Read the model definition and answer for the solid it produces. Units are mm, in the model's axes. Give positions to 0.01 mm unless a question says otherwise; leave off trailing zeros. Loops run counter-clockwise (first coordinate to the right, second up) from the corner with the lowest first, then second, coordinate; pieces in that order, holes last. Notation, with made-up numbers: M 11.5,-6 L 24.5,-6 A29 cw 24.5,24 Z; hole C 60.5,77.25 d9. An arc over 180 degrees is marked long. Return JSON: item names as keys, results as strings. Group by question number.
```python
from build123d import *

# Parameters (mm, degrees)
SKETCH1_W           = 92
SKETCH1_H           = 50
SKETCH1_R           = 10.5
SKETCH1_R_2         = 1.55
BOSS_EXTRUDE1_DEPTH = 3
FILLET1_R           = 4
SKETCH_1_R          = 3.05
CUT_EXTRUDE_1_DEPTH = 10


with BuildPart() as part:
    # Sketch1 → Boss-Extrude1 (new body)
    with BuildSketch(Plane(origin=(0, 0, 0), x_dir=(1, 0, 0), z_dir=(0, 1, 0))):
        Rectangle(SKETCH1_W, SKETCH1_H)
        with Locations(Location((0, 0, 0), (0, 0, 270))):
            Circle(SKETCH1_R, mode=Mode.SUBTRACT)
        with Locations(Location((42, 21, 0), (0, 0, 270))):
            Circle(SKETCH1_R_2, mode=Mode.SUBTRACT)
        with Locations(Location((-42, 21, 0), (0, 0, 90))):
            Circle(SKETCH1_R_2, mode=Mode.SUBTRACT)
        with Locations(Location((42, -21, 0), (0, 0, 90))):
            Circle(SKETCH1_R_2, mode=Mode.SUBTRACT)
        with Locations(Location((-42, -21, 0), (0, 0, 270))):
            Circle(SKETCH1_R_2, mode=Mode.SUBTRACT)
        with Locations(Location((0, -18, 0), (0, 0, 270))):
            Circle(SKETCH1_R_2, mode=Mode.SUBTRACT)
        with Locations(Location((-15.588457268, 9, 0), (0, 0, 270))):
            Circle(SKETCH1_R_2, mode=Mode.SUBTRACT)
        with Locations(Location((15.588457268, 9, 0), (0, 0, 270))):
            Circle(SKETCH1_R_2, mode=Mode.SUBTRACT)
    extrude(amount=BOSS_EXTRUDE1_DEPTH)

    # Fillet1
    fillet1_edges = [part.edges().sort_by_distance(p)[0] for p in [
        (46, 1.5, 25),
        (-46, 1.5, 25),
        (-46, 1.5, -25),
        (46, 1.5, -25),
    ]]
    fillet(fillet1_edges, radius=FILLET1_R)

    # 草图1 → 切除-拉伸1 (cut)
    with BuildSketch(Plane.XZ):
        with Locations(Location((-22.5, 0, 0), (0, 0, 270))):
            Circle(SKETCH_1_R)
        with Locations(Location((22.5, 0, 0), (0, 0, 270))):
            Circle(SKETCH_1_R)
    extrude(amount=-CUT_EXTRUDE_1_DEPTH, mode=Mode.SUBTRACT)


solid = part.part
```
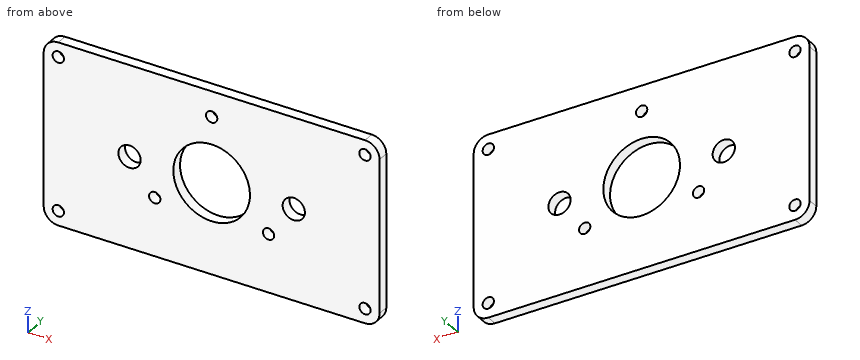
1. A flat-ended cylindrical pin translates along its axis: P1, Ø3, axis at x = 42, z = 21, coming from the +Y side. Find the tip coordinate at first contact, or state that the pin passes through.
2. Straight lines are drawn through the part: line 1 along X through (y, z) = (1.45, -21); line 2 along X through (y, z) = (1.5, -9); line 3 along X through (y, z) = (0.7, -2). For each, find the intervals that lie inside material, in ascending order.
3. Find section B-B (x = 22.5). Write down the section's boundary in (y, z), and give its area (3 significant figures).
4. Find section C-C (z = 0). Write down the section's boundary in (x, y), and give its area (3 significant figures).
5. Find section D-D (y = 0.85). State how many separate pieces and enclosed holes the cut face has, and give its area (3 significant figures).
6. Find section A-A (z = 18). Write down the section's boundary in (x, y).
Result:
{
 "1": {"P1": "passes through"},
 "2": {"line 1": "x = -46 to -43.55, -40.45 to 40.45, 43.55 to 46", "line 2": "x = -46 to -17.14, -14.04 to -5.41, 5.41 to 14.04, 17.14 to 46", "line 3": "x = -46 to -24.8, -20.2 to -10.31, 10.31 to 20.2, 24.8 to 46"},
 "3": {"outline": "M 0,-25 L 3,-25 L 3,-3.05 L 0,-3.05 Z; M 0,3.05 L 3,3.05 L 3,25 L 0,25 Z", "area": "132 mm2"},
 "4": {"outline": "M -46,0 L -25.55,0 L -25.55,3 L -46,3 Z; M -19.45,0 L -10.5,0 L -10.5,3 L -19.45,3 Z; M 10.5,0 L 19.45,0 L 19.45,3 L 10.5,3 Z; M 25.55,0 L 46,0 L 46,3 L 25.55,3 Z", "area": "176 mm2"},
 "5": {"separate pieces": "1", "enclosed holes": "10", "area": "4,130 mm2"},
 "6": {"outline": "M -46,0 L -1.55,0 L -1.55,3 L -46,3 Z; M 1.55,0 L 46,0 L 46,3 L 1.55,3 Z"}
}
